```python
from build123d import *

# Parameters (mm, degrees)
BOSS_EXTRUDE1_DEPTH = 3.175


with BuildPart() as part:
    # Sketch1 → Boss-Extrude1 (new, symmetric)
    with BuildSketch(Plane.XY):
        with BuildLine():
            Line((-553.911696572, -24.168934537), (0, -203.2))
            Line((0, -203.2), (553.911696572, -24.168934537))
            ThreePointArc((553.911696572, -24.168934537), (570.268934537, 7.811696572), (538.288303428, 24.168934537))
            Line((538.288303428, 24.168934537), (0, -149.812458319))
            Line((0, -149.812458319), (-538.288303428, 24.168934537))
            ThreePointArc((-538.288303428, 24.168934537), (-570.268934537, 7.811696572), (-553.911696572, -24.168934537))
        make_face()
    extrude(amount=BOSS_EXTRUDE1_DEPTH, both=True)


solid = part.part
```
Read the model definition and answer for the solid it produces. Units are mm, in the model's axes. A direction names the side the tool comes from. Give positions to 0.01 mm unless a question says otherwise; leave off trailing zeros. Write each loop counter-clockwise with the first axis right and the second up, starting at its lowest first coordinate (ties: lowest second). Pieces come first, ordered by that corner, then holes. Notation, with made-up numbers: (85.5, 53) - (123.5, 53) arc R13 cw to (123.5, 57) - close; hole circle Ø7 at (-6, 16.25). An arc over 180 degrees is marked (long way). Write item = value, one per line. Start each with the question number.
Item 1: Find section C-C (y = -160.5). Give the vertices of the cut face in (x, z) (3 decimals), then the cut area to 3 significant figures.
Item 2: Find section B-B (z = 0.25). Give the vertices of the cut face in (x, y), then the cut area to 3 significant figures.
Item 3: Find the intervals of material crossed by probe 1 along Y at (x, z) = (-245, 2.75); probe 2 along Y at (x, z) = (425.5, -1), in increasing order. Write a range as [from, to].
Item 4: Find section D-D (x = 233.5). Give the vertices of the cut face in (y, z) (3 decimals), then the cut area to 3 significant figures.
Item 5: Each of these flat-tipped pins is pushed along its axis until it touches: P1, Ø3, axis at x = -205.5, z = -1, coming from the -Y side; P2, Ø1, axis at x = -33.5, z = -0.5, coming from the -Y side. Where does it stop, or does it pass through?
Item 6: Find section A-A (y = -37). Give the vertices of the cut face in (x, z) (3 decimals), then the cut area to 3 significant figures.
Item 7: A tool of negligible diameter and unlimited length cuts with its end or side. For faces 1 (the flat face through (272.912, -61.604, 0.044)), 2 (the flat face through (-45, -139, 3.175)), from which of +Z, -Z, +X, -X, +Y, -Y can it reach the whole face along a straight path? Write none if from no direction.
Response:
q1.outline = (-132.111, -3.175) - (132.111, -3.175) - (132.111, 3.175) - (-132.111, 3.175) - close
q1.area = 1,680 mm²
q2.outline = (-553.91, -24.17) - (0, -203.2) - (553.91, -24.17) arc R25.4 ccw to (538.29, 24.17) - (0, -149.81) - (-538.29, 24.17) arc R25.4 ccw to start
q2.area = 60,300 mm²
q3.probe_1 = [-124.01, -70.63]
q3.probe_2 = [-65.67, -12.29]
q4.outline = (-127.73, -3.175) - (-74.342, -3.175) - (-74.342, 3.175) - (-127.73, 3.175) - close
q4.area = 339 mm²
q5.P1 = -137.26
q5.P2 = -192.53
q6.outline = (-514.213, -3.175) - (-349.035, -3.175) - (-349.035, 3.175) - (-514.213, 3.175) - close; (349.035, -3.175) - (514.213, -3.175) - (514.213, 3.175) - (349.035, 3.175) - close
q6.area = 2,100 mm²
q7.face_1 = +Z, -Z, +Y
q7.face_2 = +Z, +X, -X, +Y, -Y
